Read the model definition and answer for the solid it produces. Units are mm, in the model's axes. Coordinates: 2 decimals unless noted, no trailing zeros. Write each loop counter-clockwise with the first axis right and the second up, starting at its lowest first coordinate (ties: lowest second). Pieces come first, ordered by that corner, then holes. Notation, with made-up numbers: (-30.5, 87.5) -> (17.5, 87.5) arc R21 ccw to (17.5, 97.5) -> close; hole circle Ø1 at (53, 77.5). An arc over 180 degrees is marked (long way). Use CSV: the item, a comma, the result in double quotes.
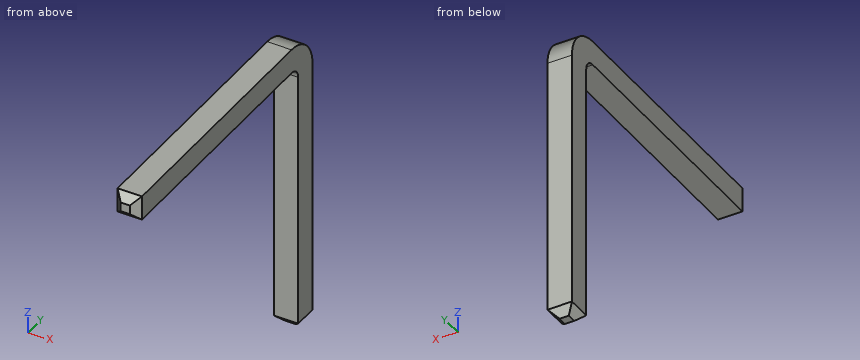
from build123d import *

# Parameters (mm, degrees)
SKETCH1_W     = 0.64
SKETCH1_H     = 0.64
CHAMFER1_SIZE = 0.2


with BuildPart() as part:
    # Sweep1: sweep along a path in Sketch2
    with BuildLine(Plane(origin=(0, 0, 0), x_dir=(0, 0, -1), z_dir=(1, 0, 0))) as sweep1_path:
        Line((0.014667815, 0), (0.014667815, 6.9))
        ThreePointArc((0.014667815, 6.9), (0.190403746, 7.324264069), (0.614667815, 7.5))
        Line((0.614667815, 7.5), (7.614667815, 7.5))
    # Sketch1 → Sweep1 (sweep)
    with BuildSketch(Plane(origin=(0, 0, 0), x_dir=(1, 0, 0), z_dir=(0, 1, 0))):
        Rectangle(SKETCH1_W, SKETCH1_H)
    sweep(path=sweep1_path.line)

    # Chamfer1
    chamfer1_edges = [part.edges().sort_by_distance(p)[0] for p in [
        (0, 0, 0.32),
        (0.32, 0, 0),
        (0, 0, -0.32),
        (-0.32, 7.514667815, -7.614667815),
        (0, 7.834667815, -7.614667815),
        (0.32, 7.514667815, -7.614667815),
        (0, 7.194667815, -7.614667815),
        (-0.32, 0, 0),
    ]]
    chamfer(chamfer1_edges, length=CHAMFER1_SIZE)


solid = part.part
1. A cutting plane is placed at B-B (z = -3). Give the vertices of the cut face in (x, y), and give its area (3 significant figures).
Solutions:
outline,"(-0.32, 7.19) -> (0.32, 7.19) -> (0.32, 7.83) -> (-0.32, 7.83) -> close"
area,"0.410 mm^2"
2. A cutting plane is placed at A-A (y = 4.5). Give the vertices of the cut face in (x, z).
Solutions:
outline,"(-0.32, -0.32) -> (0.32, -0.32) -> (0.32, 0.32) -> (-0.32, 0.32) -> close"
3. Find the intervals of material crossed by line 1 along Z through (x, y) = (-0.2, 4.25); line 2 along Y through (x, z) = (0.05, -3.5), in increasing order.
Solutions:
line 1,"z = -0.32 to 0.32"
line 2,"y = 7.19 to 7.83"
